Can you work these out from the model? Positions are in its coordinate system, mm. Face numbers are marked on the shaded views. Coordinates: 2 decimals unless noted, no trailing zeros. Order: outer loops, then holes, each group sorted by start corner. A loop starts at its lowest first (then second) coordinate and runs counter-clockwise, first axis right, second up. Notation, with made-up numbers: (77, 47.25) -> (90, 47.25) arc R9 cw to (90, 62.25) -> close; hole circle Ø5 at (0.5, -21). An arc over 180 degrees is marked (long way). Write item = value, one per line.
Autodesk Inventor part; units mm, degrees
ref_plane "YZ Plane" through (0, 0, 0) normal (1, 0, 0) x (0, 1, 0)
ref_plane "XZ Plane" through (0, 0, 0) normal (0, 1, 0) x (-1, 0, 0)
ref_plane "XY Plane" through (0, 0, 0) normal (0, 0, 1) x (1, 0, 0)
sketch "Sketch1" plane through (0, 0, 0) normal (0, 0, 1) x (1, 0, 0)
  line L0 (0, 0) -> (0, 50)
  line L1 (20, 50) -> (20, 0)
  line L2 (20, 0) -> (0, 0)
  line L3 (0, -10) -> (-48.3632, -10)
  line L4 (0, 50) -> (4.0958, 47.1321)
  line L5 (20, 50) -> (15.9042, 47.1321)
  line L6 (4.0958, 47.1321) -> (15.9042, 47.1321)
  dimension "d3" = 10
revolve "Revolution1" add sketch "Sketch1" angle 360 about axis through (0, -10, 0) along (-1, 0, 0)
thicken "Thicken1" operation add thickness 3 both sides no extend neighbours no toward (-1, 0, 0) faces at (0, -50.5351, 14.7961)
thicken "Thicken2" operation add thickness 3 both sides no extend neighbours no toward (1, 0, 0) faces at (20, -50.5351, -14.7961)
sketch "Sketch2" plane through (-3, -10, 0) normal (-1, 0, 0) x (0, 0, 1)
  line L0 (-3.5, 5) -> (3.5, 5)
  line L1 (3.5, 5) -> (3.5, 15)
  line L2 (3.5, 15) -> (-3.5, 15)
  line L3 (-3.5, 15) -> (-3.5, 5)
  line L4 (-3.5, 5) -> (3.5, 15) construction
  line L5 (3.5, 5) -> (-3.5, 15) construction
  point P0 (0, 10)
  dimension "d11" = 7
  dimension "d12" = 10
extrude "Extrusion1" cut sketch "Sketch2" against normal through all
properties part number "POLEA"
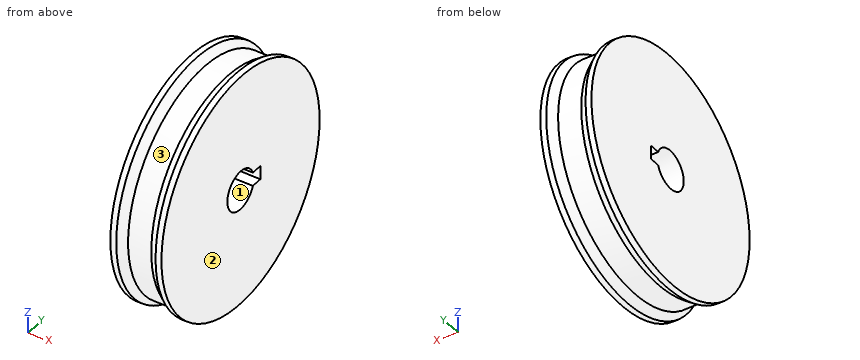
Item 1: If I drill on probe 1 along Y at (x, z) = (13.25, 0); probe 2 along Z at (x, y) = (7.75, -10); probe 3 along Z at (x, y) = (14.5, -16.5), over which ranges is the centre line in solid material (lowest first)?
A:
probe_1 = -67.13 to -20, 5 to 47.13
probe_2 = -57.13 to -10, 10 to 57.13
probe_3 = -56.76 to -7.6, 7.6 to 56.76
Item 2: If we mould it in two halves opening along Y, with no side actions, what happens to the marked faces 1, 2 and 3? For each: pulls with the +Y half, pulls with the -Y half, needs draft (parallel to the pull), parting line crosses it, or undercut.
A:
face_1 = undercut
face_2 = needs draft
face_3 = parting line crosses it
Item 3: I'm going to push flat-ended pins straight in: P1, Ø1.5, axis at x = 18.5, y = 27.5, coming from the +Z side; P2, Ø8, axis at x = 1, y = -46.5, coming from the -Z side; P3, Ø6, axis at x = 16.5, y = 2, coming from the +Z side; P4, Ø16, axis at y = -10, z = 0, coming from the +X side. Where does each tip first touch, or does it pass through?
A:
P1 = 46.39
P2 = -50.35
P3 = 58.51
P4 = through
Item 4: I want a section at A-A, the plane z = 0. Please give me the cut outline in (x, y), plus the area to 3 significant figures.
A:
outline = (-3, -70) -> (0, -70) -> (4.1, -67.13) -> (15.9, -67.13) -> (20, -70) -> (23, -70) -> (23, -20) -> (-3, -20) -> close; (-3, 5) -> (23, 5) -> (23, 50) -> (20, 50) -> (15.9, 47.13) -> (4.1, 47.13) -> (0, 50) -> (-3, 50) -> close
area = 2,380 mm2
Item 5: I want a section at C-C, the plane x = 18.25. Please give me the cut outline in (y, z).
A:
outline = circle Ø117.55 at (-10, 0); hole (-0.63, -3.5) -> (5, -3.5) -> (5, 3.5) -> (-0.63, 3.5) arc R10 ccw (long way) to start
Item 6: I want a section at B-B, the plane y = -10. Please give me the cut outline in (x, z).
A:
outline = (-3, -60) -> (0, -60) -> (4.1, -57.13) -> (15.9, -57.13) -> (20, -60) -> (23, -60) -> (23, -10) -> (-3, -10) -> close; (-3, 10) -> (23, 10) -> (23, 60) -> (20, 60) -> (15.9, 57.13) -> (4.1, 57.13) -> (0, 60) -> (-3, 60) -> close
